Here's how the part is built. I have some questions about the finished solid (model axes, mm). Coordinates: 2 decimals unless noted, no trailing zeros. Write each loop counter-clockwise with the first axis right and the second up, starting at its lowest first coordinate (ties: lowest second). Pieces come first, ordered by that corner, then holes. Notation, with made-up numbers: (-29, 66) - (22, 66) arc R24 cw to (22, 78) - close; hole circle Ø11 at (-31, 45.25). An arc over 180 degrees is marked (long way). Answer in a Markdown table with one row per item. Add a question column.
Item 1: Imagine slicing it at D-D (x = 62.5). Please give me the cut outline in (y, z) (3 decimals), plus the area to 3 significant figures.
Item 2: If I drill on probe 1 along Z at (x, y) = (80.5, 1.65); probe 2 along X at (y, z) = (3.05, -45) (3 decimals); probe 3 along X at (y, z) = (0.85, -60), over which ranges is the centre line in solid material (lowest first)? Write a range as from..to.
Item 3: We'd pull the mould along Z, two halves only. Please class faces 1 (the face through (181.305, 1.61, -41.865)), 2 (the face through (100, 3.175, -65)): +Z half, -Z half, draft (parallel to the pull), parting line (faces both ways), or undercut.
Item 4: Imagine slicing it at A-A (z = -44.45). Please give me the cut outline in (x, y) (1 decimal), plus the area to 3 significant figures.
Item 5: Imagine slicing it at B-B (x = 96). Please give me the cut outline in (y, z) (3 decimals), plus the area to 3 significant figures.
Item 6: Imagine slicing it at C-C (z = -57). Please give me the cut outline in (x, y) (3 decimals), plus the area to 3 significant figures.
Item 7: I'm going to push flat-ended pins straight in: pin 1 (1.6 mm diameter, centred on y = 2, z = -18.5, fed in from -X) (3 decimals); pin 2 (1 mm diameter, centred on x = 1.5, y = 1, fed in from -Z); pin 3 (2 mm diameter, centred on x = 55.118, z = -72.009, fed in from +Y). Where does each tip first touch, or does it pass through?
from build123d import *

# Parameters (mm, degrees)
SKETCH1_W             = 203.2
SKETCH1_H             = 88.9
BOSS_EXTRUDE1_DEPTH   = 3.175
SKETCH2_W             = 31.75
SKETCH2_H             = 8.128
SKETCH2_W_2           = 3.175
SKETCH2_H_2           = 12.7
SKETCH2_W_3           = 12.7
SKETCH2_W_4           = 38.1
CUT_EXTRUDE1_DEPTH    = 222.818688629
SKETCH3_W             = 97.028
SKETCH3_H             = 39.878
SKETCH3_W_2           = 42.926
SKETCH3_H_2           = 7.112
CUT_EXTRUDE2_DEPTH    = 222.818688629
M3_CLEARANCE_HOLE1_D  = 3.4
M12_CLEARANCE_HOLE1_D = 13.5


with BuildPart() as part:
    # Sketch1 → Boss-Extrude1 (new body)
    with BuildSketch(Plane(origin=(0, 0, 0), x_dir=(1, 0, 0), z_dir=(0, 1, 0))):
        with Locations((101.6, 44.45)):
            Rectangle(SKETCH1_W, SKETCH1_H)
    extrude(amount=BOSS_EXTRUDE1_DEPTH)

    # Sketch2 → Cut-Extrude1 (cut, through all)
    with BuildSketch(Plane(origin=(0, 3.175, 0), x_dir=(1, 0, 0), z_dir=(0, 1, 0))):
        with Locations((15.875, 84.836)):
            Rectangle(SKETCH2_W, SKETCH2_H)
        with Locations((1.5875, 44.45)):
            Rectangle(SKETCH2_W_2, SKETCH2_H_2)
        with Locations((1.5875, 69.85)):
            Rectangle(SKETCH2_W_2, SKETCH2_H_2)
        with Locations((1.5875, 19.05)):
            Rectangle(SKETCH2_W_2, SKETCH2_H_2)
        with Locations((50.8, 84.836)):
            Rectangle(SKETCH2_W_3, SKETCH2_H)
        with Locations((88.9, 84.836)):
            Rectangle(SKETCH2_W_4, SKETCH2_H)
        with Locations((127, 84.836)):
            Rectangle(SKETCH2_W_3, SKETCH2_H)
        with Locations((152.4, 84.836)):
            Rectangle(SKETCH2_W_3, SKETCH2_H)
        with Locations((187.325, 84.836)):
            Rectangle(SKETCH2_W, SKETCH2_H)
        with Locations((201.6125, 19.05)):
            Rectangle(SKETCH2_W_2, SKETCH2_H_2)
        with Locations((201.6125, 44.45)):
            Rectangle(SKETCH2_W_2, SKETCH2_H_2)
        with Locations((201.6125, 69.85)):
            Rectangle(SKETCH2_W_2, SKETCH2_H_2)
    extrude(amount=-CUT_EXTRUDE1_DEPTH, mode=Mode.SUBTRACT)

    # Sketch3 → Cut-Extrude2 (cut, through all)
    with BuildSketch(Plane.XZ):
        with Locations((101.6, -44.45)):
            Rectangle(SKETCH3_W, SKETCH3_H)
        with Locations((80.645, -71.755)):
            Rectangle(SKETCH3_W_2, SKETCH3_H_2)
    extrude(amount=-CUT_EXTRUDE2_DEPTH, mode=Mode.SUBTRACT)

    # M3 Clearance Hole1 (through all)
    with Locations(Plane(origin=(0, 0, 0), x_dir=(-1, 0, 0), z_dir=(0, -1, 0))):
        with Locations((-148.082, 72.009), (-148.082, 16.891), (-55.118, 16.891), (-55.118, 72.009)):
            Hole(M3_CLEARANCE_HOLE1_D / 2)

    # M12 Clearance Hole1 (through all)
    with Locations(Plane(origin=(0, 0, 0), x_dir=(-1, 0, 0), z_dir=(0, -1, 0))):
        with Locations((-175.0695, 44.45), (-28.1305, 44.45)):
            Hole(M12_CLEARANCE_HOLE1_D / 2)


solid = part.part
Here are the results:
| question | item | result |
|---|---|---|
| 1 | outline | (0, -88.9) - (3.175, -88.9) - (3.175, -75.311) - (0, -75.311) - close; (0, -68.199) - (3.175, -68.199) - (3.175, -64.389) - (0, -64.389) - close; (0, -24.511) - (3.175, -24.511) - (3.175, 0) - (0, 0) - close |
| 1 | area | 133 mm2 |
| 2 | probe 1 | z = -80.77..-75.31, -68.2..-64.39, -24.51..0 |
| 2 | probe 2 | x = 3.175..21.403, 34.858..53.086, 150.114..168.342, 181.797..200.025 |
| 2 | probe 3 | x = 0..53.09, 150.11..203.2 |
| 3 | face 1 | undercut |
| 3 | face 2 | draft |
| 4 | outline | (3.2, 0) - (21.4, 0) - (21.4, 3.2) - (3.2, 3.2) - close; (34.9, 0) - (53.1, 0) - (53.1, 3.2) - (34.9, 3.2) - close; (150.1, 0) - (168.3, 0) - (168.3, 3.2) - (150.1, 3.2) - close; (181.8, 0) - (200, 0) - (200, 3.2) - (181.8, 3.2) - close |
| 4 | area | 231 mm2 |
| 5 | outline | (0, -80.772) - (3.175, -80.772) - (3.175, -75.311) - (0, -75.311) - close; (0, -68.199) - (3.175, -68.199) - (3.175, -64.389) - (0, -64.389) - close; (0, -24.511) - (3.175, -24.511) - (3.175, 0) - (0, 0) - close |
| 5 | area | 107 mm2 |
| 6 | outline | (0, 0) - (53.086, 0) - (53.086, 3.175) - (0, 3.175) - close; (150.114, 0) - (203.2, 0) - (203.2, 3.175) - (150.114, 3.175) - close |
| 6 | area | 337 mm2 |
| 7 | pin 1 | stops at x = 3.175 |
| 7 | pin 2 | stops at z = -80.77 |
| 7 | pin 3 | passes through |
